Can you work these out from the model? Positions are in its coordinate system, mm. A direction names the side the tool comes from. Give positions to 0.01 mm unless a question says otherwise; leave off trailing zeros. Loops run counter-clockwise (first coordinate to the right, second up) from the corner with the lowest first, then second, coordinate; pieces in that order, holes last. Notation, with made-up numbers: M 6,20 L 32,20 A13 ccw 32,45 Z; hole C 20.5,22 d5. An arc over 180 degrees is marked long. Put each result on its own line as item: value. Start each with the question number.
1) Please list where these lines run through material, in increasing order: line 1 along Y through (x, z) = (0, 2.5); line 2 along X through (y, z) = (-14, 5.5); line 3 along X through (y, z) = (-41.5, 4). Write a range as from..to.
2) Imagine slicing it at C-C (y = -19). Write out the boundary of the cut face in (x, z), then the cut area to 3 significant figures.
3) If we mould it in two halves opening along X, with no side actions, what happens to faces 5 (the flat face through (21, -10, 0)), 6 (the cylindrical face through (-17.897, -22.632, 4.418))? For each: +X half, -X half, draft (parallel to the pull), parting line (faces both ways), or undercut.
4) For P1, Ø5.5, axis at x = -35.08, y = 0, coming from the +Z side; P2, Ø3, axis at y = -28, z = 2.5, coming from the +X side; P3, Ø2, axis at y = -25.5, z = 3.5, coming from the +X side; P4, Ø1.5, axis at y = 2.5, z = 2.5, coming from the +X side, each with a flat end and sliding along its axis, tell me the tip position at first contact or that it passes through.
5) For faces 1 (the flat face through (-17.9, -12.4, 6.35)), 2 (the flat face through (4.71, 46.26, 3.13)), 3 (the flat face through (-4.86, 46.46, 3.13)), 4 (the cylindrical face through (31.72, -22.63, 4.42)), which set-ups out of +Z, -Z, +X, -X, +Y, -Y let a thin tool reach every point of the face, with its end or its side?
6) Imagine slicing it at A-A (y = 0). State how many separate pieces and enclosed holes the cut face has, then the cut area to 3 significant figures.
7) Imagine slicing it at D-D (y = 10). Write out the boundary of the cut face in (x, z), then the cut area to 3 significant figures.
from build123d import *

# Parameters (mm, degrees)
F0_R        = 4.7064707614
F0_R_2      = 21.5186597363
F1_DEPTH    = 6.35
F2_T        = 2.54
F2_T3_DEPTH = 11.43


# Not quite as in the source:
# - a shell that OpenCascade refuses in one call is made with other operations: the cavity is built on its own and cut out


with BuildPart() as f1:
    # F0 (on Top) → F1 (new body)
    with BuildSketch(Plane.XY):
        with BuildLine():
            Line((-4.9161130278, 45.3357483006), (-4.8021092029, 47.6136840266))
            ThreePointArc((-4.8021092029, 47.6136840266), (0.0120888652, -47.8552297376), (4.7780528964, 47.6161041025))
            Line((4.7780528964, 47.6161041025), (4.639992765, 44.8574939765))
            Line((4.639992765, 44.8574939765), (-0.2761202627, 42.3380110126))
            Line((-0.2761202627, 42.3380110126), (-4.9161130278, 45.3357483006))
        make_face()
        with Locations((-24.80855963, -24.80855963)):
            Circle(F0_R, mode=Mode.SUBTRACT)
        with Locations((0, -35.0846014917)):
            Circle(F0_R, mode=Mode.SUBTRACT)
        with Locations((24.80855963, -24.80855963)):
            Circle(F0_R, mode=Mode.SUBTRACT)
        with Locations((-35.0846014917, 0)):
            Circle(F0_R, mode=Mode.SUBTRACT)
        with Locations((-24.80855963, 24.80855963)):
            Circle(F0_R, mode=Mode.SUBTRACT)
        Circle(F0_R_2, mode=Mode.SUBTRACT)
        with Locations((35.0846014917, 0)):
            Circle(F0_R, mode=Mode.SUBTRACT)
        with Locations((0, 35.0846014917)):
            Circle(F0_R, mode=Mode.SUBTRACT)
        with Locations((24.80855963, 24.80855963)):
            Circle(F0_R, mode=Mode.SUBTRACT)
    extrude(amount=F1_DEPTH)

    # F2: shell of thickness 2.54, made by hand


with BuildPart() as f2_core1:
    # F2_t2: copy of F1
    add(f1.part)

    # the walls: a layer under each face that stays
    f2_faces = [f2_core1.faces().sort_by_distance(p)[0] for p in [
        (-2.5961166453, 43.8368796566, 3.175),
        (-4.8591111154, 46.4747161636, 3.175),
        (0.0120888652, -47.8552297376, 3.175),
        (4.7090228307, 46.2367990395, 3.175),
        (2.1819362512, 43.5977524946, 3.175),
        (-29.5150303914, -24.80855963, 3.175),
        (-4.7064707614, -35.0846014917, 3.175),
        (20.1020888686, -24.80855963, 3.175),
        (-39.7910722531, 0, 3.175),
        (-29.5150303914, 24.80855963, 3.175),
        (-21.5186597363, 0, 3.175),
        (30.3781307302, 0, 3.175),
        (-4.7064707614, 35.0846014917, 3.175),
        (20.1020888686, 24.80855963, 3.175),
        (-31.9034875097, -31.9433420367, 0),
    ]]
    thicken(f2_faces, amount=-F2_T, mode=Mode.SUBTRACT)

    # F2_s4 → F2_t3 (cut)
    with BuildSketch(Plane.XY.offset(-2.54)):
        Polygon((-0.2739212432, 42.3819501104), (-1.6544837368, 40.2045363506), (-0.4227215664, 39.4087378278), (0.8823412559, 40.0775758974), align=None)
        Polygon((-4.8769611431, 45.3558134427), (-6.2944765018, 43.2022736386), (-7.5262386722, 43.9980721614), (-7.4529380204, 45.4627087538), align=None)
        Polygon((4.6030398999, 44.8813679322), (7.1768177577, 44.7305335234), (7.1035171059, 43.265896931), (5.7984542836, 42.5970588614), align=None)
    extrude(amount=F2_T3_DEPTH, mode=Mode.SUBTRACT)


with BuildPart() as f1_1:
    add(f1.part)

    # what is left inside the walls is the cavity
    f2_cavity = [f2_core1.part.solids().sort_by_distance(p)[0] for p in [
        (-22.657616, 14.723726, 2.5654),
    ]]
    add(f2_cavity, mode=Mode.SUBTRACT)


solid = f1_1.part
Recorded:
1. line 1: -47.86..-39.79, -30.38..-21.52, 21.52..30.38, 39.79..42.48
1. line 2: -45.76..-43.1, -19.57..-16.34, 16.34..19.57, 43.1..45.76
1. line 3: -23.83..-18.2, -3.37..3.37, 18.2..23.83
2. outline: M -43.92,0 L -10.1,0 L -10.1,6.35 L -14.76,6.35 L -14.76,2.54 L -20.48,2.54 L -20.48,6.35 L -29.14,6.35 L -29.14,2.54 L -41.14,2.54 L -41.14,6.35 L -43.92,6.35 Z; M 10.1,0 L 43.92,0 L 43.92,6.35 L 41.14,6.35 L 41.14,2.54 L 29.14,2.54 L 29.14,6.35 L 20.48,6.35 L 20.48,2.54 L 14.76,2.54 L 14.76,6.35 L 10.1,6.35 Z
2. area: 295 mm²
3. face 5: draft
3. face 6: undercut
4. P1: through
4. P2: x = 39.85
4. P3: x = 41.11
4. P4: x = 47.82
5. face 1: +Z, +X, -X, +Y, -Y
5. face 2: +Z, -Z, +Y
5. face 3: +Z, -Z
5. face 4: +Z
6. separate pieces: 4
6. enclosed holes: 0
6. area: 163 mm²
7. outline: M -46.8,0 L -19.05,0 L -19.05,6.35 L -21.88,6.35 L -21.88,2.54 L -44.2,2.54 L -44.2,6.35 L -46.8,6.35 Z; M 19.05,0 L 46.8,0 L 46.8,6.35 L 44.2,6.35 L 44.2,2.54 L 21.88,2.54 L 21.88,6.35 L 19.05,6.35 Z
7. area: 182 mm²
